Drawing for the job (mm, zero at the part's lowest x, y, z). A direction names the side the tool comes from. Coordinates: 2 decimals unless noted, no trailing zeros. Write each loop counter-clockwise with the first axis right and the second up, starting at its lowest first coordinate (ties: lowest second). Pieces come first, ordered by that corner, then holes. Notation, with made-up numbers: (62, 82.25) -> (74, 82.25) arc R18 cw to (74, 97.25) -> close; hole circle Ø1 at (15, -27.5). An arc over 180 degrees is marked (long way). Write item = value, one per line. Start each with the question number.
Q1. Band-saw the part on A-A, the plane y = 5.25. List the corners of the cut face in (x, z).
Q2. Pull direction X, two halves, no side cores. Call the marked faces 4, 5 and 6: released by +X, released by -X, zero draft, split by the parting line, or undercut.
Q3. Probe line 1 (Y direction, x = 68.5, z = 10); line 2 (Y direction, x = 29.5, z = 21.5); line 3 (X direction, y = 17.25, z = 10.75). List the from-to ranges inside material, lowest first.
Q4. Band-saw the part on C-C, the plane y = 11.75. List the corners of the cut face in (x, z).
Q5. Tool access for the marked faces 1, 2 and 3: list every direction of +Z, -Z, +X, -X, +Y, -Y with a clear straight run to the whole face (end or side of a thin tool).
Q6. Band-saw the part on B-B, the plane x = 53.5. List the corners of the cut face in (y, z).
Q7. Pin check, flat tips, straight feed: P1, Ø2, axis at x = 8, z = 16.5, coming from the +Y side; P2, Ø1.4, axis at x = 81.5, z = 18, coming from the -Y side; P3, Ø1.5, axis at x = 54, z = 22, coming from the +Y side. Stop position of each tip, or through.
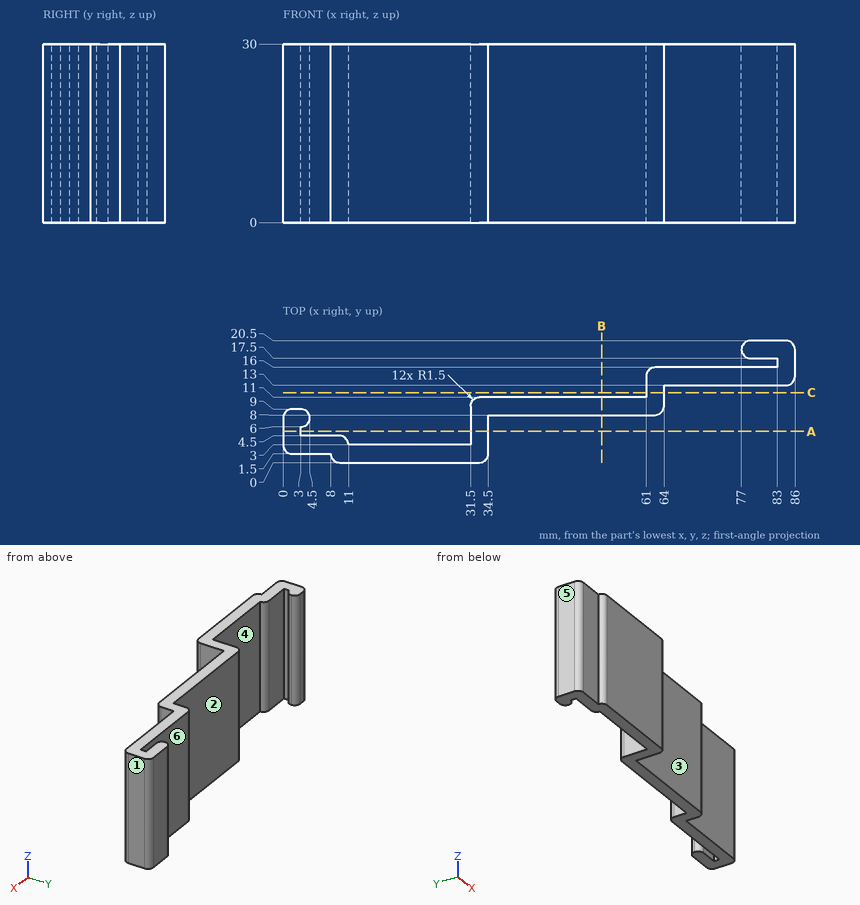
Ans:
q1.outline = (0, 0) -> (3, 0) -> (3, 30) -> (0, 30) -> close; (31.5, 0) -> (34.5, 0) -> (34.5, 30) -> (31.5, 30) -> close
q2.face_4 = undercut
q2.face_5 = released by -X
q2.face_6 = zero draft
q3.line_1 = 13 to 16
q3.line_2 = 0 to 3
q3.line_3 = 83 to 86
q4.outline = (61, 0) -> (64, 0) -> (64, 30) -> (61, 30) -> close
q5.face_1 = +Z, -Z, +X, +Y, -Y
q5.face_2 = +Z, -Z, -X, +Y
q5.face_3 = +Z, -Z, +X, -Y
q6.outline = (8, 0) -> (11, 0) -> (11, 30) -> (8, 30) -> close
q7.P1 = 4.5
q7.P2 = 13
q7.P3 = 11
